Geometry: final body of the model. Coordinates: model frame, mm. A direction names the side the tool comes from. Give positions to 0.01 mm unless a question says otherwise; leave off trailing zeros. Order: outer loops, then holes, each group sorted by start corner. A loop starts at its lowest first (then second) coordinate and runs counter-clockwise, first axis right, second up. Notation, with made-up numbers: (14.25, 38.5) - (31.25, 38.5) arc R17 ccw to (31.25, 42.5) - close; hole circle Ø8 at (-16, 0.5). An arc over 180 degrees is marked (long way). Put each result on its own line as item: value. Start each with the question number.
1. First-contact query: P1, Ø12.5, axis at x = -35.5, z = 1, coming from the +Y side; P2, Ø5, axis at x = 24.5, y = -9.5, coming from the +Z side; P3, Ø2, axis at y = -14.5, z = -2, coming from the -X side. Flat tips, straight axial feed; report the tip coordinate or a pass-through.
2. Section D-D on x = -21.5. Return the cut outline in (y, z).
3. Set-up query: faces 1 (the flat face through (6, -8, 8)), 2 (the flat face through (5, -8, -8)), 3 (the flat face through (-31, -9, 0)), 4 (the flat face through (39, -8, 0)). Return all of +Z, -Z, +X, -X, +Y, -Y with unobstructed straight access to the full face (end or side cutting, diameter ignored); none if empty.
4. Section A-A on z = 0. Return the cut outline in (x, y).
5. Ray query, line 1 along Z through (x, y) = (46, -1.75); line 2 along Z through (x, y) = (-28.5, -15); line 3 along Y through (x, z) = (-43, 9). Return the intervals inside material, ascending. Write a range as from..to.
6. Section C-C on y = -13. Return the cut outline in (x, z), plus the area to 3 significant figures.
7. Mould query, pull axis Z, two halves, no side actions, for faces 5 (the cylindrical face through (-33.354, -12.944, -2.298)), 6 (the cylindrical face through (56.1, -3.9, -0.3)), 7 (the cylindrical face through (51.646, -3.944, -2.298)), 8 (the flat face through (38, 0, 0)). Classes: pulls with the +Z half, pulls with the -Z half, needs draft (parallel to the pull), parting line crosses it, or undercut.
8. Section B-B on x = 42.5. Return the cut outline in (y, z).
from build123d import *

# Parameters (mm, degrees)
F0_R     = 6
F1_DEPTH = 25
F3_DEPTH = 12.5


with BuildPart() as f1:
    # F0 (on Front) → F1 (new body)
    with BuildSketch(Plane.XZ):
        with BuildLine():
            Line((40.103297, 8), (-29.292017, 8))
            ThreePointArc((-29.292017, 8), (-51.396703, 0), (-29.292017, -8))
            Line((-29.292017, -8), (40.103297, -8))
            ThreePointArc((40.103297, -8), (56.103297, 0), (40.103297, 8))
        make_face()
        with Locations((-38.896703, 0)):
            Circle(F0_R, mode=Mode.SUBTRACT)
        with Locations((46.103297, 0)):
            Circle(F0_R, mode=Mode.SUBTRACT)
    extrude(amount=F1_DEPTH)

    # F2 (on Top) → F3 (intersect, symmetric)
    with BuildSketch(Plane.XY):
        Polygon((-19.159218, -9), (-51.396703, -9), (-51.396703, -17), (-18.459309, -17), (32.582227, -8), (56.103297, -8), (56.103297, 0), (31.882318, 0), align=None)
    extrude(amount=F3_DEPTH, both=True, mode=Mode.INTERSECT)


solid = f1.part
Resolved:
1. P1: y = -9
1. P2: z = 8
1. P3: x = -51.36
2. outline: (-17, -8) - (-9, -8) - (-9, 8) - (-17, 8) - close
3. face 1: +Z, +Y, -Y
3. face 2: -Z, +Y, -Y
3. face 3: +Z, -Z, -X, +Y
3. face 4: +Z, -Z, +X, -Y
4. outline: (-51.4, -17) - (-44.9, -17) - (-44.9, -9) - (-51.4, -9) - close; (-32.9, -17) - (-18.46, -17) - (32.58, -8) - (40.1, -8) - (40.1, 0) - (31.88, 0) - (-19.16, -9) - (-32.9, -9) - close; (52.1, -8) - (56.1, -8) - (56.1, 0) - (52.1, 0) - close
5. line 1: -10..-6, 6..10
5. line 2: -8..8
5. line 3: -17..-9
6. outline: (-29.29, -8) - (4.23, -8) - (4.23, 8) - (-29.29, 8) arc R12.5 ccw (long way) to start; hole circle Ø12 at (-38.9, 0)
6. area: 882 mm^2
7. face 5: undercut
7. face 6: parting line crosses it
7. face 7: undercut
7. face 8: needs draft
8. outline: (-8, -9.33) - (0, -9.33) - (0, -4.8) - (-8, -4.8) - close; (-8, 4.8) - (0, 4.8) - (0, 9.33) - (-8, 9.33) - close
